Autodesk Inventor part; units mm, degrees
ref_plane "Work Plane1" through (30, 0, 0) normal (1, 0, 0) x (0, 1, 0)
ref_plane "XZ Plane" through (0, 0, 0) normal (0, 1, 0) x (-1, 0, 0)
ref_plane "XY Plane" through (0, 0, 0) normal (0, 0, 1) x (1, 0, 0)
sketch "Sketch1" plane through (0, 0, 0) normal (0, 0, 1) x (1, 0, 0)
  line L0 (0, 0) -> (60, 0)
  line L1 (60, 0) -> (60, 40)
  line L2 (60, 40) -> (0, 40)
  line L3 (0, 40) -> (0, 0)
extrude "Extrusion1" add sketch "Sketch1" along normal blind 10
sketch "Sketch2" plane through (0, 0, 0) normal (0, 0, 1) x (1, 0, 0)
  line L0 (7, 7) -> (13, 7)
  line L1 (13, 7) -> (13, 13)
  line L2 (13, 13) -> (7, 13)
  line L3 (7, 13) -> (7, 7)
extrude "Extrusion2" cut sketch "Sketch2" along normal blind 10
ref_plane "Work Plane1" through (30, 0, 0) normal (1, 0, 0) x (0, 1, 0)
mirror "Mirror1" about plane through (30, 0, 0) normal (1, 0, 0) of "Extrusion2"
properties part number "23_pocket_mirror"
For this review, take the finished solid that the model builds, in its own axes (mm). A direction names the side the tool comes from. Coordinates: 2 decimals unless noted, no trailing zeros. Loops run counter-clockwise (first coordinate to the right, second up) from the corner with the lowest first, then second, coordinate; pieces in that order, holes last. Notation, with made-up numbers: (-8.75, 16.5) - (30.25, 16.5) arc R29 cw to (30.25, 47.5) - close; hole circle Ø5 at (26.25, 62.25). An arc over 180 degrees is marked (long way). Use one line per item in the form item = value. Start each with the question number.
1) Take a section at B-B (x = 9). State the section outline as (y, z) points, plus the area to 3 significant figures.
2) Take a section at A-A (y = 10). State the section outline as (x, z) points.
3) For faces 4 (the face through (30, 40, 5)), 5 (the face through (50, 13, 5)), list the 3-axis set-ups (+Z, -Z, +X, -X, +Y, -Y) from which the entire face can be reached by the end or side of a thin tool; tool diameter is ignored.
4) To check wall thickness, follow probe 1 along X at (y, z) = (11, 8.25); probe 2 along Y at (x, z) = (10.5, 4). State the ranges of each line that lie inside material, in increasing order. Write a range as from..to.
5) Take a section at C-C (z = 5.75). State the section outline as (x, y) points, plus the area to 3 significant figures.
6) Draft analysis for pull direction X (two halves, no side actions). For faces 1 (the face through (30, 20, 10)), 2 (the face through (7, 10, 5)), 3 (the face through (0, 20, 5)), state which applies: released by +X, released by -X, zero draft, split by the parting line, or undercut.
From the geometry:
q1.outline = (0, 0) - (7, 0) - (7, 10) - (0, 10) - close; (13, 0) - (40, 0) - (40, 10) - (13, 10) - close
q1.area = 340 mm2
q2.outline = (0, 0) - (7, 0) - (7, 10) - (0, 10) - close; (13, 0) - (47, 0) - (47, 10) - (13, 10) - close; (53, 0) - (60, 0) - (60, 10) - (53, 10) - close
q3.face_4 = +Z, -Z, +X, -X, +Y
q3.face_5 = +Z, -Z
q4.probe_1 = 0..7, 13..47, 53..60
q4.probe_2 = 0..7, 13..40
q5.outline = (0, 0) - (60, 0) - (60, 40) - (0, 40) - close; hole (7, 7) - (13, 7) - (13, 13) - (7, 13) - close; hole (47, 7) - (53, 7) - (53, 13) - (47, 13) - close
q5.area = 2,330 mm2
q6.face_1 = zero draft
q6.face_2 = undercut
q6.face_3 = released by -X
